Verification items for this drawing (mm, ordinates from the low corner). Coordinates: 2 decimals unless noted, no trailing zeros. Order: outer loops, then holes, each group sorted by start corner. A loop starts at its lowest first (then second) coordinate and runs counter-clockwise, first axis right, second up. Notation, with made-up numbers: (16.25, 20.5) -> (20.25, 20.5) arc R8 cw to (20.25, 26.5) -> close; hole circle Ø4 at (60.25, -3.75). An arc over 180 degrees is marked (long way). Put each result on its own line as item: value. Start each with the question number.
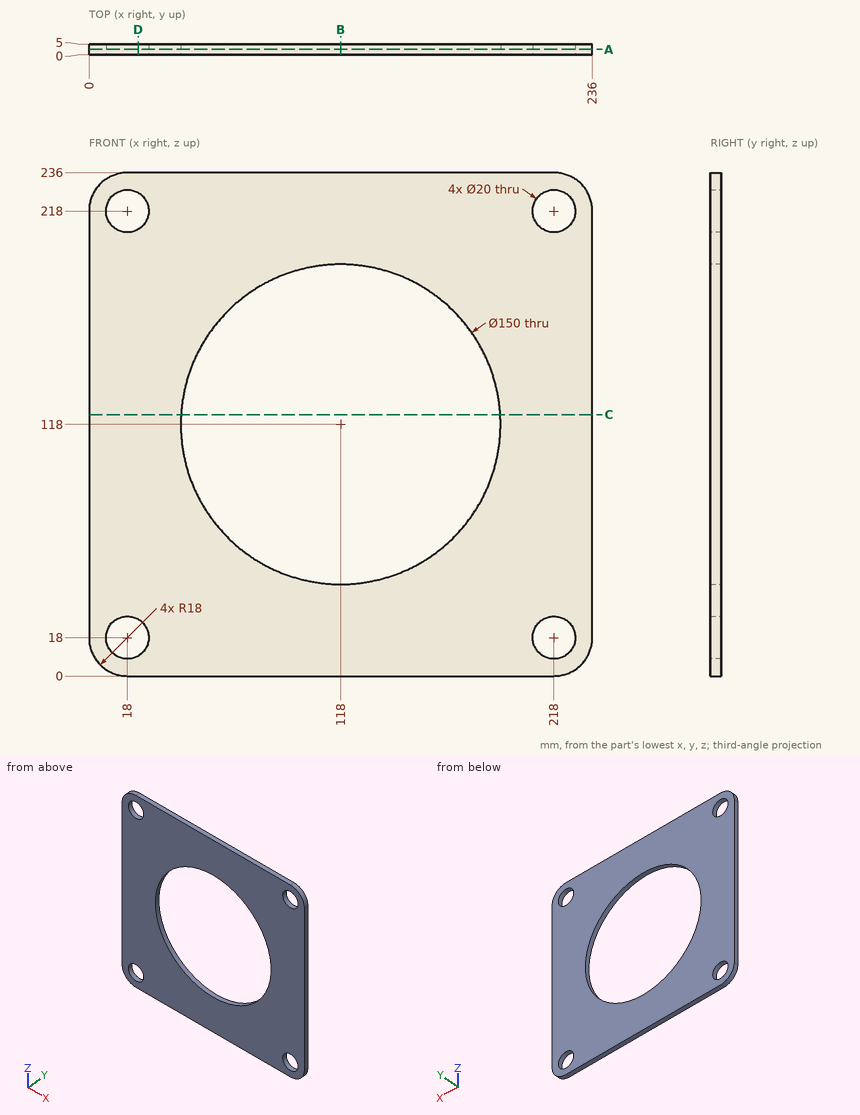
1) Sectioned sample at A-A (y = 2.5). Record the boundary of the cut face in (x, z).
2) Scan lines: line 1 along X through (y, z) = (3.7, 218); line 2 along X through (y, z) = (0.85, 211); line 3 along Z through (x, y) = (87.5, 2.85). Record each from-to range of solid material in increasing order. Write a range as [from, to].
3) Sectioned sample at B-B (x = 118). Record the boundary of the cut face in (y, z), plus the area to 3 significant figures.
4) Sectioned sample at C-C (z = 122.5). Record the boundary of the cut face in (x, y).
5) Sectioned sample at D-D (x = 23). Record the boundary of the cut face in (y, z), plus the area to 3 significant figures.
Entries:
1. outline: (0, 18) arc R18 ccw to (18, 0) -> (218, 0) arc R18 ccw to (236, 18) -> (236, 218) arc R18 ccw to (218, 236) -> (18, 236) arc R18 ccw to (0, 218) -> close; hole circle Ø20 at (18, 18); hole circle Ø20 at (18, 218); hole circle Ø150 at (118, 118); hole circle Ø20 at (218, 18); hole circle Ø20 at (218, 218)
2. line 1: x = [0, 8], [28, 208], [228, 236]
2. line 2: x = [0, 10.86], [25.14, 210.86], [225.14, 236]
2. line 3: z = [0, 49.48], [186.52, 236]
3. outline: (0, 0) -> (5, 0) -> (5, 43) -> (0, 43) -> close; (0, 193) -> (5, 193) -> (5, 236) -> (0, 236) -> close
3. area: 430 mm2
4. outline: (0, 0) -> (43.14, 0) -> (43.14, 5) -> (0, 5) -> close; (192.86, 0) -> (236, 0) -> (236, 5) -> (192.86, 5) -> close
5. outline: (0, 0) -> (5, 0) -> (5, 9.34) -> (0, 9.34) -> close; (0, 26.66) -> (5, 26.66) -> (5, 209.34) -> (0, 209.34) -> close; (0, 226.66) -> (5, 226.66) -> (5, 236) -> (0, 236) -> close
5. area: 1,010 mm2
